from build123d import *

# Parameters (mm, degrees)
SKETCH1_W                        = 40
SKETCH1_H                        = 70
BOSS_EXTRUDE1_DEPTH              = 59
SKETCH2_R                        = 11
SKETCH2_R_2                      = 2.5
CUT_EXTRUDE1_DEPTH               = 72.504101247
SKETCH5_R                        = 2.5
CUT_EXTRUDE3_DEPTH               = 5
TAP_DRILL_FOR_M5_HELICOIL1_D     = 5.2
TAP_DRILL_FOR_M5_HELICOIL1_DEPTH = 6.437762391
TAP_DRILL_FOR_M5_HELICOIL1_TIP   = 1.562237609


with BuildPart() as part:
    # Sketch1 → Boss-Extrude1 (new body)
    with BuildSketch(Plane.XY):
        with Locations((0.060830656, 0.062794648)):
            Rectangle(SKETCH1_W, SKETCH1_H)
    extrude(amount=BOSS_EXTRUDE1_DEPTH)

    # Sketch2 → Cut-Extrude1 (cut, through all)
    with BuildSketch(Plane.XY):
        Circle(SKETCH2_R)
        with Locations((-11.313708499, 11.313708499)):
            Circle(SKETCH2_R_2)
        with Locations((-0.122338904, 15.759725587)):
            Circle(SKETCH2_R_2)
        with Locations((11.402693442, 11.263696484)):
            Circle(SKETCH2_R_2)
        with Locations((11.339369089, -11.406422087)):
            Circle(SKETCH2_R_2)
        with Locations((-0.312311964, -16.029099896)):
            Circle(SKETCH2_R_2)
        with Locations((-11.204100775, -11.406422087)):
            Circle(SKETCH2_R_2)
    extrude(amount=CUT_EXTRUDE1_DEPTH, mode=Mode.SUBTRACT)

    # Sketch5 → Cut-Extrude3 (cut)
    with BuildSketch(Plane.ZY.offset(19.939169344)):
        with Locations((29.5, 0.062794648)):
            Circle(SKETCH5_R)
        with Locations((39.5, 0.062794648)):
            Circle(SKETCH5_R)
        with Locations((19.5, 0.062794648)):
            Circle(SKETCH5_R)
        with Locations((29.5, 10.062794648)):
            Circle(SKETCH5_R)
        with Locations((29.5, -9.937205352)):
            Circle(SKETCH5_R)
    extrude(amount=-CUT_EXTRUDE3_DEPTH, mode=Mode.SUBTRACT)

    # Tap Drill for M5 Helicoil1
    with Locations(Plane(origin=(20.060830656, 0, 0), x_dir=(0, 0, -1), z_dir=(1, 0, 0))):
        with Locations((-52.500633733, 6.530017119), (-52.500633733, -6.469982881), (-6.500633733, -6.469982881), (-6.500633733, 6.530017119)):
            Hole(TAP_DRILL_FOR_M5_HELICOIL1_D / 2, depth=TAP_DRILL_FOR_M5_HELICOIL1_DEPTH)
            with Locations((0, 0, -(TAP_DRILL_FOR_M5_HELICOIL1_DEPTH + TAP_DRILL_FOR_M5_HELICOIL1_TIP / 2))):  # 118° drill point
                Cone(0, TAP_DRILL_FOR_M5_HELICOIL1_D / 2, TAP_DRILL_FOR_M5_HELICOIL1_TIP, mode=Mode.SUBTRACT)


solid = part.part
Check sheet for the modelled part. Datum: model origin and axes. Units: mm. A direction names the side the tool comes from. Give positions to 0.01 mm unless a question says otherwise; leave off trailing zeros. Write each loop counter-clockwise with the first axis right and the second up, starting at its lowest first coordinate (ties: lowest second). Pieces come first, ordered by that corner, then holes. Notation, with made-up numbers: (-31, -36.5) -> (-17, -36.5) arc R20 ccw to (-17, -20.5) -> close; hole circle Ø7 at (-32.5, -22.75). An arc over 180 degrees is marked (long way). Use one line per item in the form item = value. Start each with the question number.
1. Section check C-C (z = 34.5). Record the cut outline in (x, y), and give its area (3 significant figures).
2. Thickness scan on line 1 along Z through (x, y) = (16.5, 6.5); line 2 along X through (y, z) = (-12.5, 15); line 3 along Y through (x, z) = (12, 49.5). Record the ranges inside material, lowest first. Write a range as from..to.
3. Access from +Z, -Z, +X, -X, +Y, -Y to the whole of each face (thin tool, end or side, straight path). Record for faces 1 (the flat face through (-14.939, 0, 39)), 2 (the flat face through (20.061, 0, 29)), 3 (the cylindrical face through (16.797, 4.223, 7.7)).
4. Mould release check, pull along Y, two halves, no side actions. Record for faces 4 (the flat face through (9, 8, 59)), 5 (the cylindrical face through (16.8, 6.6, 49.9)): pulls with the +Y half, pulls with the -Y half, needs draft (parallel to the pull), parting line crosses it, or undercut.
5. Go/stop test with flat-tipped pins: P1, Ø2.5, axis at y = 0.5, z = 40, coming from the -X side; P2, Ø3, axis at y = -6.47, z = 6.5, coming from the +X side; P3, Ø4.5, axis at y = -6.47, z = 52.5, coming from the +X side. Record where each tip stops, or that it passes through.
6. Section check A-A (x = 0). Record the cut outline in (y, z), and give its area (3 significant figures).
7. Section check D-D (x = -17). Record the cut outline in (y, z).
8. Section check B-B (x = -4). Record the cut outline in (y, z).
Conclusion:
q1.outline = (-19.94, -34.94) -> (20.06, -34.94) -> (20.06, 35.06) -> (-19.94, 35.06) -> close; hole circle Ø5 at (-11.31, 11.31); hole circle Ø5 at (-11.2, -11.41); hole circle Ø22 at (0, 0); hole circle Ø5 at (-0.31, -16.03); hole circle Ø5 at (-0.12, 15.76); hole circle Ø5 at (11.34, -11.41); hole circle Ø5 at (11.4, 11.26)
q1.area = 2,300 mm²
q2.line_1 = 0..3.9, 9.1..49.9, 55.1..59
q2.line_2 = -19.94..-13.45, -8.96..9.09, 13.59..20.06
q2.line_3 = -34.94..-13.82, -9..8.84, 13.69..35.06
q3.face_1 = -X
q3.face_2 = +Z, -Z, +X, +Y, -Y
q3.face_3 = +X
q4.face_4 = needs draft
q4.face_5 = undercut
q5.P1 = -14.94
q5.P2 = 12.96
q5.P3 = 13.41
q6.outline = (-34.94, 0) -> (-18.51, 0) -> (-18.51, 59) -> (-34.94, 59) -> close; (-13.55, 0) -> (-11, 0) -> (-11, 59) -> (-13.55, 59) -> close; (11, 0) -> (13.26, 0) -> (13.26, 59) -> (11, 59) -> close; (18.26, 0) -> (35.06, 0) -> (35.06, 59) -> (18.26, 59) -> close
q6.area = 2,240 mm²
q7.outline = (-34.94, 0) -> (35.06, 0) -> (35.06, 59) -> (-34.94, 59) -> close; hole circle Ø5 at (-9.94, 29.5); hole circle Ø5 at (0.06, 19.5); hole circle Ø5 at (0.06, 29.5); hole circle Ø5 at (0.06, 39.5); hole circle Ø5 at (10.06, 29.5)
q8.outline = (-34.94, 0) -> (-10.25, 0) -> (-10.25, 59) -> (-34.94, 59) -> close; (10.25, 0) -> (35.06, 0) -> (35.06, 59) -> (10.25, 59) -> close
